Autodesk Inventor part; units mm, degrees
ref_plane "YZ Plane" through (0, 0, 0) normal (1, 0, 0) x (0, 1, 0)
ref_plane "XZ Plane" through (0, 0, 0) normal (0, 1, 0) x (-1, 0, 0)
ref_plane "XY Plane" through (0, 0, 0) normal (0, 0, 1) x (1, 0, 0)
ref_plane "Work Plane1" through (0, 0, 0) normal (0, 0, 1) x (1, 0, 0)
sketch "Sketch1" plane through (0, 0, 0) normal (0, 0, 1) x (1, 0, 0)
  line L0 (374.65, 19.755) -> (374.65, -0.245)
  line L1 (394.65, -0.245) -> (394.65, 19.755)
  line L2 (374.65, -0.245) -> (394.65, -0.245)
  line L3 (374.65, -0.245) -> (372.11, -0.245)
  line L4 (372.11, -0.245) -> (372.11, 19.755)
  line L5 (372.11, 19.755) -> (374.65, 19.755)
  line L6 (374.65, 19.755) -> (374.65, -0.245)
  line L7 (372.11, 19.755) -> (394.65, 19.755)
  line L8 (394.65, 19.755) -> (394.65, 24.835)
  line L9 (394.65, 24.835) -> (372.11, 24.835)
  line L10 (372.11, 24.835) -> (372.11, 19.755)
  point P0 (0, 0)
  dimension "d0" = 2.54
  dimension "d1" = 20
  dimension "d2" = 5.08
extrude "Extrusion1" add sketch "Sketch1" along normal mid plane 20 contours L0 L3 L4 L5 | L5 L10 L9 L8 L7
sketch "Sketch2" plane through (372.11, 24.835, -10) normal (0, 1, 0) x (1, 0, 0)
  line L0 (0, 0) -> (22.54, 0)
  line L1 (0, 0) -> (0, -20)
  line L2 (22.54, -20) -> (0, -20)
  line L3 (22.54, 0) -> (22.54, -20)
  line L4 (2.54, -340.2) -> (2.54, 320.2)
  line L5 (2.54, -20) -> (2.54, 0)
  line L6 (2.54, -10) -> (22.54, -10)
  circle A0 centre (12.54, -10) radius 2.5
  point P0 (-372.11, -10)
  dimension "d5" = 5
extrude "Extrusion2" cut sketch "Sketch2" against normal blind 20 contours A0 L6 | L6 A0
sketch "Sketch3" plane through (374.65, -0.245, -10) normal (1, 0, 0) x (0, 0, -1)
  line L0 (0, 20) -> (0, 0)
  line L1 (0, 20) -> (-20, 20)
  circle A0 centre (-10, 10) radius 2.5
  point P0 (-10, 0.245)
  dimension "d8" = 5
extrude "Extrusion3" cut sketch "Sketch3" against normal blind 20
sketch "Sketch4" plane through (0, 0, -10) normal (0, 0, -1) x (-1, 0, 0)
  line L0 (-374.65, -0.245) -> (-374.65, 19.755)
  line L1 (-374.65, 19.755) -> (-394.65, 19.755)
  line L2 (-394.65, 19.755) -> (-394.65, 24.835)
  line L3 (-394.65, 24.835) -> (-372.11, 24.835)
  line L4 (-372.11, 24.835) -> (-372.11, -0.245)
  line L5 (-372.11, -0.245) -> (-374.65, -0.245)
  line L6 (-372.11, -0.245) -> (-330.11, -0.245)
  line L7 (-330.11, -0.245) -> (-330.11, 41.755)
  line L8 (-330.11, 41.755) -> (-372.11, 41.755)
  line L9 (-372.11, 41.755) -> (-372.11, -0.245)
  circle A0 centre (-351.11, 20.755) radius 12.5
  circle A1 centre (-335.61, 36.255) radius 2
  circle A2 centre (-335.61, 5.255) radius 2
  circle A3 centre (-366.61, 36.255) radius 2
  circle A4 centre (-366.61, 5.255) radius 2
  point P0 (0, 0)
  dimension "d11" = 42
  dimension "d12" = 42
  dimension "d13" = 25
  dimension "d16" = 4
  dimension "d19" = 31
  dimension "d22" = 31
extrude "Extrusion4" add sketch "Sketch4" along normal blind 5.08
chamfer "Chamfer1" distance 16.764 angle 45 1 edges at (372.11, 24.835, -12.54)
properties part number "YMotorMount"
The listing builds one solid part. Answer for the finished solid, in the listing's coordinates (mm). A direction names the side the tool comes from. Round coordinates to 2 decimals unless told otherwise and drop trailing zeros. Order: outer loops, then holes, each group sorted by start corner. A loop starts at its lowest first (then second) coordinate and runs counter-clockwise, first axis right, second up. Notation, with made-up numbers: (29.25, -24.5) -> (75.25, -24.5) arc R7 ccw to (75.25, -16.5) -> close; hole circle Ø8 at (29.5, -31.5). An arc over 180 degrees is marked (long way). Answer as CSV lines item,"result". Start each with the question number.
(1) Find the intervals of material crossed by probe 1 along Y at (x, z) = (366.61, -11.7) (3 decimals); probe 2 along Z at (x, y) = (376.5, 28); probe 3 along X at (y, z) = (8, 3.75), in increasing order. Write a range as from..to.
(2) The part is cut by section A-A (x = 335.61). Determine the outline of the cut face in (y, z) (3 decimals).
(3) The part is cut by section B-B (y = 23.5). Determine the outline of the cut face in (x, z), then the cut area to 3 significant figures.
(4) A tool of negligible diameter and unlimited length cuts with its end or side. For faces 1 (the face through (385, 19.755, -3)), 2 (the face through (360, 30, -10)), 3 (the face through (330.11, 20, -13)), from which of +Z, -Z, +X, -X, +Y, -Y can it reach the whole face along a straight path? Write none if from no direction.
(5) For a pull along Y with two mould halves and no side action, classify faces 4 (the face through (372.11, 12, 2)), 5 (the face through (384, 24.835, -3)), 6 (the face through (356, -0.245, -11)), 7 (the face through (333.702, 4.654, -12.504)) as +Y half, -Y half, draft (parallel to the pull), parting line (faces both ways), or undercut.
(6) The part is cut by section D-D (y = 13.5). Determine the outline of the cut face in (x, z), then the cut area to 3 significant figures.
(7) The part is cut by section C-C (x = 351.11). Determine the outline of the cut face in (y, z) (3 decimals).
(8) Flat-ended cylindrical pins translate along their axes: pin 1 Ø6.5 at (x, y) = (366.61, 5.255) entering from +Z; pin 2 Ø5 at (x, z) = (367, -7) entering from +Y; pin 3 Ø6 at (x, z) = (378, 3) entering from +Y (3 decimals); pin 4 Ø8 at (x, z) = (384.65, 0) entering from -Y (3 decimals). Find the tip coordinate at first contact, or state that the pin passes through.
Evaluation:
1,probe 1,"-0.245..3.255, 7.255..34.255, 38.255..41.755"
1,probe 2,"-15.08..-10"
1,probe 3,"372.11..374.65"
2,outline,"(-0.245, -15.08) -> (3.255, -15.08) -> (3.255, -10) -> (-0.245, -10) -> close; (7.255, -15.08) -> (34.255, -15.08) -> (34.255, -10) -> (7.255, -10) -> close; (38.255, -15.08) -> (41.755, -15.08) -> (41.755, -10) -> (38.255, -10) -> close"
3,outline,"(330.11, -15.08) -> (338.92, -15.08) -> (338.92, -10) -> (330.11, -10) -> close; (363.3, -15.08) -> (394.65, -15.08) -> (394.65, 10) -> (372.11, 10) -> (372.11, -10) -> (363.3, -10) -> close; hole circle Ø5 at (384.65, 0)"
3,area,"635 mm²"
4,face 1,"+Z, -Z, +X, -Y"
4,face 2,"+Z, -X, +Y"
4,face 3,"+Z, -Z, -X, +Y, -Y"
5,face 4,"draft"
5,face 5,"+Y half"
5,face 6,"-Y half"
5,face 7,"undercut"
6,outline,"(330.11, -15.08) -> (340.93, -15.08) -> (340.93, -10) -> (330.11, -10) -> close; (361.29, -15.08) -> (374.65, -15.08) -> (374.65, 10) -> (372.11, 10) -> (372.11, -10) -> (361.29, -10) -> close"
6,area,"174 mm²"
7,outline,"(-0.245, -15.08) -> (8.255, -15.08) -> (8.255, -10) -> (-0.245, -10) -> close; (33.255, -15.08) -> (41.755, -15.08) -> (41.755, -10) -> (33.255, -10) -> close"
8,pin 1,"z = -10"
8,pin 2,"through"
8,pin 3,"y = 24.835"
8,pin 4,"y = 19.755"
